Design review of the part built by this model. Coordinates are the model's own, in mm. Give positions to 0.01 mm unless a question says otherwise; leave off trailing zeros. Loops run counter-clockwise (first coordinate to the right, second up) from the corner with the lowest first, then second, coordinate; pieces in that order, holes last. Notation, with made-up numbers: M -25,-25 L 20,-25 A21 cw 20,5 Z; hole C 58.25,-20 d7. An arc over 180 degrees is marked long. Use CSV: the item, a comma, the result in double quotes.
from build123d import *

# Parameters (mm, degrees)
SKETCH3_R           = 1.5
BOSS_EXTRUDE1_DEPTH = 5
SKETCH4_R           = 1
CUT_EXTRUDE1_DEPTH  = 8.04531685
FILLET1_R           = 0.5
SCALE_1_SCALE       = 0.894736842


with BuildPart() as part:
    # Sketch2 → Revolve2 (revolve)
    with BuildSketch(Plane(origin=(0, 0, 0), x_dir=(0, 0, -1), z_dir=(1, 0, 0))):
        with BuildLine():
            Line((0, 1.54531685), (0, 0))
            Line((0, 0), (0, -0.5))
            Line((0, -0.5), (-3.730724896, -0.5))
            Line((-3.730724896, -0.5), (-3.730724896, 0))
            ThreePointArc((-3.730724896, 0), (-2.019053765, 1.143702085), (0, 1.54531685))
        make_face()
    revolve(axis=Axis((0, -0.5, 0), (0, 1, 0)))

    # Sketch3 → Boss-Extrude1 (add)
    with BuildSketch(Plane.XZ.offset(0.5)):
        Circle(SKETCH3_R)
    extrude(amount=BOSS_EXTRUDE1_DEPTH)

    # Sketch4 → Cut-Extrude1 (cut, through all)
    with BuildSketch(Plane.XZ.offset(5.5)):
        Circle(SKETCH4_R)
    extrude(amount=-CUT_EXTRUDE1_DEPTH, mode=Mode.SUBTRACT)

    # Fillet1
    fillet1_edges = [part.edges().sort_by_distance(p)[0] for p in [
        (-0.707106781, 1.449682086, -0.707106781),
    ]]
    fillet(fillet1_edges, radius=FILLET1_R)


with BuildPart() as part_1:
    # ｽｹｰﾙ1: scaled about (5.91e-07, -0.705292116, -1.889e-06)
    add(part.part.scale(SCALE_1_SCALE).moved(Location((6.2e-08, -0.074241275, -1.99e-07))))


solid = part_1.part
(1) We need section C-C on x = -2.5. State the section outline as (y, z) points, then the cut area to 3 significant figures.
A:
outline,"M -0.52,-2.21 L -0.07,-2.21 A4 ccw -0.07,2.21 L -0.52,2.21 Z"
area,"3.98 mm²"
(2) We need section D-D on y = 0.5. State the section outline as (x, z) points, then the cut area to 3 significant figures.
A:
outline,"C 0,0 d5.28; hole C 0,0 d1.79"
area,"19.4 mm²"
(3) We need section B-B on z = 2.75. State the section outline as (x, y) points, then the cut area to 3 significant figures.
A:
outline,"M -1.89,-0.52 L 1.89,-0.52 L 1.89,-0.07 A3.84 ccw -1.89,-0.07 Z"
area,"2.97 mm²"
(4) We need section A-A on y = -4.25. State the section outline as (x, z) points, then the cut area to 3 significant figures.
A:
outline,"C 0,0 d2.68; hole C 0,0 d1.79"
area,"3.14 mm²"
(5) Wall thickness on line 1 along X through (y, z) = (-1.85, 0); line 2 along X through (y, z) = (-1.5, 1): over which ranges is each line inside the solid? List them lowest first. Write a range as [from, to].
A:
line 1,"[-1.34, -0.89], [0.89, 1.34]"
line 2,"[-0.9, 0.9]"
(6) Clearance check with a flat-ended pin moving along its axis: P1, Ø1.6, axis at x = 0, z = 0, coming from the -Y side. State where the tip first meets the part, or that it passes through.
A:
P1,"through"
(7) The part is to be moulded in two halves that separate along X. For faces 1 (the cylindrical face through (3.31, -0.29, -0.43)), 2 (the cylindrical face through (0.853, -2.215, 0.269)), 3 (the flat face through (-1.4, -0.522, -0.7)), say which applies: released by +X, released by -X, zero draft, split by the parting line, or undercut.
A:
face 1,"split by the parting line"
face 2,"undercut"
face 3,"zero draft"
